Work out the finished part from the listing and answer in its coordinate system (mm). Face numbers are marked on the shaded views. A direction names the side the tool comes from. Coordinates: 2 decimals unless noted, no trailing zeros. Order: outer loops, then holes, each group sorted by start corner. A loop starts at its lowest first (then second) coordinate and runs counter-clockwise, first axis right, second up. Notation, with made-up numbers: M 24.25,77 L 38.25,77 A12 ccw 38.25,98 Z; hole C -11.75,-9.75 d1. An arc over 180 degrees is marked long. Use a Markdown table: item, result.
from build123d import *

# Parameters (mm, degrees)
F0_R     = 500
F1_DEPTH = 1100
F2_R     = 200
F3_R     = 194.129707
F3_R_2   = 178.794503
F4_DEPTH = 160


with BuildPart() as f1:
    # F0 (on Top) → F1 (new body)
    with BuildSketch(Plane.XY):
        Circle(F0_R)
    extrude(amount=F1_DEPTH)

    # F2
    f2_edges = [f1.edges().sort_by_distance(p)[0] for p in [
        (-500, 0, 0),
        (-500, 0, 1100),
    ]]
    fillet(f2_edges, radius=F2_R)

    # F3 (on face) → F4 (join)
    with BuildSketch(Plane.XY.offset(1100)):
        Circle(F3_R)
        Circle(F3_R_2, mode=Mode.SUBTRACT)
    extrude(amount=F4_DEPTH)


solid = f1.part
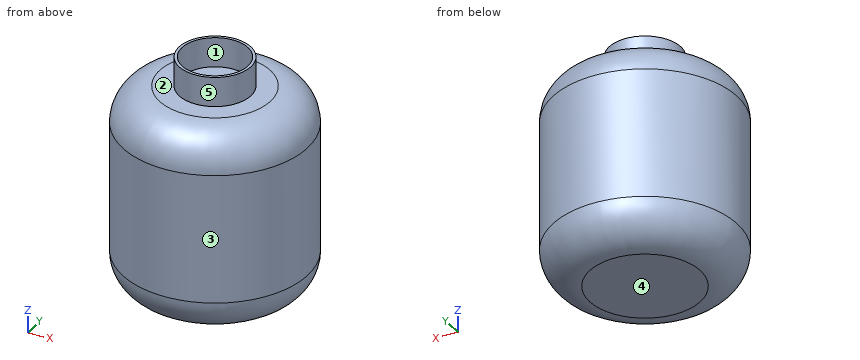
(1) Straight lines are drawn through the part: L1, parallel to Y at x = 0, z = 1166; L2, parallel to Z at x = -236.5, y = 53; L3, parallel to X at y = -339, z = 638.5. For each, find the intervals that lie inside material, in ascending order.
Conclusion:
| item | result |
|---|---|
| L1 | -194.13 to -178.79, 178.79 to 194.13 |
| L2 | 0 to 1100 |
| L3 | -367.53 to 367.53 |
(2) Which of the six approach directions +Z, -Z, +X, -X, +Y, -Y give full straight-line access (tool end or side, diameter ignored) to the marked faces 4 and 5?
Conclusion:
| item | result |
|---|---|
| face 4 | -Z, +X, -X, +Y, -Y |
| face 5 | +Z |
(3) A cutting plane is placed at C-C (z = 824.5). Determine the outline of the cut face in (x, y).
Conclusion:
| item | result |
|---|---|
| outline | C 0,0 d1000 |
(4) A cutting plane is placed at D-D (z = 142). Determine the outline of the cut face in (x, y), then the cut area to 3 significant figures.
Conclusion:
| item | result |
|---|---|
| outline | C 0,0 d982.81 |
| area | 759,000 mm2 |
(5) Given P1, Ø8, axis at y = -264.5, z = 441, coming from the -X side; P2, Ø2, axis at x = 156.5, z = 692, coming from the +Y side; P3, Ø10, axis at y = -139.5, z = 573, coming from the +X side, each flat-ended and moving along its own axis, determine where each tip first touches the part or whether it passes through.
Conclusion:
| item | result |
|---|---|
| P1 | x = -426.78 |
| P2 | y = 475.2 |
| P3 | x = 481.57 |
(6) A cutting plane is placed at A-A (x = 0). Determine the outline of the cut face in (y, z).
Conclusion:
| item | result |
|---|---|
| outline | M -500,200 A200 ccw -300,0 L 300,0 A200 ccw 500,200 L 500,900 A200 ccw 300,1100 L 194.13,1100 L 194.13,1260 L 178.79,1260 L 178.79,1100 L -178.79,1100 L -178.79,1260 L -194.13,1260 L -194.13,1100 L -300,1100 A200 ccw -500,900 Z |
(7) Determine the mould class of the marked faces 1, 2 and 3 for opening direction X: pulls with the +X half, pulls with the -X half, needs draft (parallel to the pull), parting line crosses it, or undercut.
Conclusion:
| item | result |
|---|---|
| face 1 | undercut |
| face 2 | needs draft |
| face 3 | parting line crosses it |
